For this review, take the finished solid that the model builds, in its own axes (mm). A direction names the side the tool comes from. Give positions to 0.01 mm unless a question says otherwise; leave off trailing zeros. Order: outer loops, then holes, each group sorted by start corner. A loop starts at its lowest first (then second) coordinate and runs counter-clockwise, first axis right, second up. Notation, with made-up numbers: M 11,-34.75 L 27,-34.75 A26 ccw 27,-20.75 Z; hole C 68,57 d7. An arc over 180 degrees is marked long. Answer as CSV lines item,"result". Start each with the question number.
1. We need section A-A, the plane z = 2. Give the boundary of the cut face in (x, y).
2. Clearance check with flat-ended pins moving along their axes: P1, Ø4, axis at y = -2, z = -0.5, coming from the +X side; P2, Ø1, axis at y = -8, z = 10, coming from the -X side; P3, Ø1.5, axis at x = 33.5, y = -5.5, coming from the -Z side. State where each tip first meets the part, or that it passes through.
3. We need section B-B, the plane y = 15.5. Give the boundary of the cut face in (x, z), and give its area (3 significant figures).
4. For line 1 along Y through (x, z) = (20, 19.5); line 2 along X through (y, z) = (7.5, 6); line 3 along Z through (x, y) = (29, -2), list the stretches that pass through material, from the lowest coordinate up.
5. Machinability: for faces 5 (the flat face through (26, 10, 18)), 6 (the flat face through (8.75, -7, 7)), 7 (the flat face through (34, 0, 15)), 8 (the cylindrical face through (12.63, 6.51, 19.45)), 9 (the flat face through (26, -10, 18)), which of the approach directions +Z, -Z, +X, -X, +Y, -Y give a long, thin tool a straight path to every point of the face, cutting with its end or side? Answer none if there is none.
6. Mouldability with a two-part tool opening along X and no side actions: class faces 1 (the cylindrical face through (18.389, -0.14, 14.625)), 2 (the flat face through (23.75, 0, 25)), 3 (the flat face through (43.75, 0, 21)), 4 (the flat face through (0, 25, 0)) as pulls with the +X half, pulls with the -X half, needs draft (parallel to the pull), parting line crosses it, or undercut.
from build123d import *

# Parameters (mm, degrees)
F1_DEPTH = 25
F0_W     = 10
F0_H     = 7.5
F0_H_2   = 1.88
F0_H_3   = 1.87
F2_DEPTH = 10
F3_DEPTH = 3.125


with BuildPart() as f1:
    # F0 (on Front) → F1 (new body, symmetric)
    with BuildSketch(Plane.XZ):
        Polygon((16.25, -3.75), (16.25, 3.75), (8.75, 3.75), (-16.25, 3.75), (-16.25, -3.75), align=None)
    extrude(amount=F1_DEPTH, both=True)

    # F0 (on Front) → F2 (join, symmetric)
    with BuildSketch(Plane.XZ):
        with BuildLine():
            Line((8.75, 3.75), (16.25, 3.75))
            Line((16.25, 3.75), (16.25, 9.38))
            ThreePointArc((16.25, 9.38), (18.4466991411, 14.6833008589), (23.75, 16.88))
            Line((23.75, 16.88), (23.75, 24.38))
            add(Edge.make_bspline(
                [(21.9670846153, 24.2736635094), (22.5617558007, 24.3196900172), (23.156226413, 24.3552224615), (23.75, 24.38)],
                knots=[43.3513201218, 43.3513201218, 43.3513201218, 43.3513201218, 45.0066317336, 45.0066317336, 45.0066317336, 45.0066317336], degree=3))
            ThreePointArc((21.9670846153, 24.2736635094), (12.5307368609, 19.3363112956), (8.75, 9.38))
            Line((8.75, 9.38), (8.75, 3.75))
        make_face()
        with Locations((28.75, 20.63)):
            Rectangle(F0_W, F0_H)
        with Locations((28.75, 15.94)):
            Rectangle(F0_W, F0_H_2)
        with Locations((28.75, 25.315)):
            Rectangle(F0_W, F0_H_3)
        Polygon((33.75, 24.38), (33.75, 16.88), (33.75, 15), (43.75, 15), (43.75, 26.25), (33.75, 26.25), align=None)
    extrude(amount=F2_DEPTH, both=True)

    # F0 (on Front) → F3 (join, symmetric)
    with BuildSketch(Plane.XZ):
        with BuildLine():
            Line((-16.25, 3.75), (8.75, 3.75))
            Line((8.75, 3.75), (8.75, 9.38))
            ThreePointArc((8.75, 9.38), (12.5307368609, 19.3363112956), (21.9670846153, 24.2736635094))
            add(Edge.make_bspline(
                [(-16.25, 3.75), (-9.3184325712, 14.665248361), (6.3931100598, 23.0682651661), (21.9670846153, 24.2736635094)],
                knots=[0, 0, 0, 0, 43.3513201218, 43.3513201218, 43.3513201218, 43.3513201218], degree=3))
        make_face()
    extrude(amount=F3_DEPTH, both=True)


solid = f1.part
Result set:
1,outline,"M -16.25,-25 L 16.25,-25 L 16.25,25 L -16.25,25 Z"
2,P1,"x = 16.25"
2,P2,"x = 8.75"
2,P3,"z = 15"
3,outline,"M -16.25,-3.75 L 16.25,-3.75 L 16.25,3.75 L -16.25,3.75 Z"
3,area,"244 mm2"
4,line 1,"-10 to 10"
4,line 2,"8.75 to 16.25"
4,line 3,"15 to 26.25"
5,face 5,"+Z, +X, -X, +Y"
5,face 6,"+Z, -X, -Y"
5,face 7,"-Z, +X, +Y, -Y"
5,face 8,"+Z, -X, +Y"
5,face 9,"+Z, +X, -X, -Y"
6,face 1,"undercut"
6,face 2,"pulls with the -X half"
6,face 3,"pulls with the +X half"
6,face 4,"needs draft"
